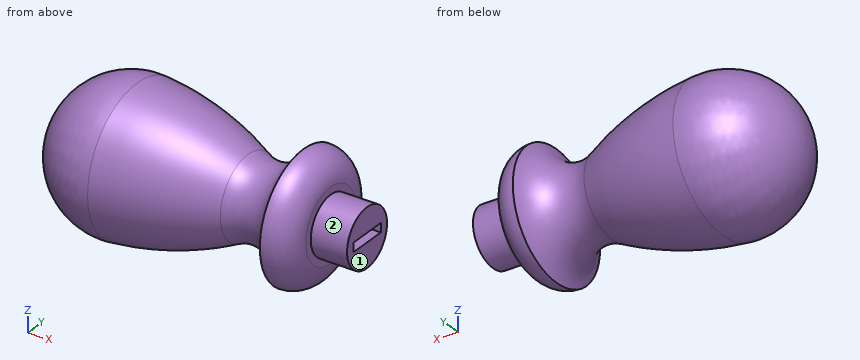
```python
from build123d import *

# Parameters (mm, degrees)
F2_W     = 11
F2_H     = 2.5
F3_DEPTH = 55


with BuildPart() as f1:
    # F0 (on Front) → F1 (revolve)
    with BuildSketch(Plane.XZ):
        with BuildLine():
            ThreePointArc((32.263173, 11.182035), (17.416574, 17.027463), (1.726048, 19.92538))
            ThreePointArc((1.726048, 19.92538), (-13.518118, 14.739759), (-20, 0))
            Line((-20, 0), (0, 0))
            Line((0, 0), (65, 0))
            Line((65, 0), (65, 8))
            Line((65, 8), (55, 8))
            Line((55, 8), (55, 10))
            ThreePointArc((55, 10), (52.803301, 15.303301), (47.5, 17.5))
            ThreePointArc((47.5, 17.5), (41.338742, 10.826844), (32.263173, 11.182035))
        make_face()
    revolve(axis=Axis((32.5, 0, 0), (1, 0, 0)))

    # F2 (on face) → F3 (cut)
    with BuildSketch(Plane.YZ.offset(65)):
        Rectangle(F2_W, F2_H)
    extrude(amount=-F3_DEPTH, mode=Mode.SUBTRACT)


solid = f1.part
```
Part model, mm, in its own coordinate system. Face numbers are marked on the shaded views. A direction names the side the tool comes from. Round coordinates to 2 decimals unless told otherwise and drop trailing zeros. Loops run counter-clockwise (first coordinate to the right, second up) from the corner with the lowest first, then second, coordinate; pieces in that order, holes last.
Item 1: Drill centre lines: line 1 (X direction, y = -12.5, z = 1); line 2 (X direction, y = -9, z = 13); line 3 (Y direction, x = 13.5, z = 0). Where is each one in solid material? Low to high.
Item 2: 3-axis set-ups, long thin cutter, end or side, ignore diameter. For the marked faces 1 and 2: which of +Z, -Z, +X, -X, +Y, -Y reach the whole face in a straight line?
Item 3: Cut at A-A, the plane x = 36. Give the cut face in (y, z), then the cut area to 3 significant figures.
Item 4: Drop flat-ended pins along their axis: P1, Ø6, axis at y = 14, z = 7.5, coming from the +X side; P2, Ø2, axis at x = 49, z = 0.5, coming from the -Y side; P3, Ø1.5, axis at x = 1, z = -1, coming from the +Y side; P4, Ø2, axis at y = -0.5, z = 0.5, coming from the +X side. Give the stop position or say it passes through.
A:
1. line 1: x = -15.58 to 29.47, 44.16 to 54.56
1. line 2: x = -12.25 to 21.3, 46.79 to 52.24
1. line 3: y = -18.05 to -5.5, 5.5 to 18.05
2. face 1: +Z, -Z, +X, +Y, -Y
2. face 2: +X
3. outline: circle Ø20.13 at (0, 0); hole (-5.5, -1.25) - (5.5, -1.25) - (5.5, 1.25) - (-5.5, 1.25) - close
3. area: 291 mm2
4. P1: stops at x = 54.42
4. P2: stops at y = -17.48
4. P3: stops at y = 19.99
4. P4: stops at x = 65
